from build123d import *
from build123d.topology import SkipClean

# Parameters (mm, degrees)
SKETCH_1_R               = 2.05
EXTRUDE_1_DEPTH          = 3
EXTRUDE_START            = -3
SKETCH_2_R               = 2.05
SKETCH_2_R_2             = 1.65
SKETCH_2_R_3             = 6
EXTRUDE_2_DEPTH          = 3
SKETCH_3_R               = 4
EXTRUDE_3_DEPTH          = 2
EXTRUDE_4_DEPTH          = 1.5
SKETCH_5_R               = 12.75
SKETCH_5_R_2             = 10.75
EXTRUDE_5_DEPTH          = 20
CUT_EXTRUDE_START        = -3
SKETCH_6_R               = 10.75
CUT_EXTRUDE_1_DEPTH      = 3
SKETCH_8_R               = 12.75
SKETCH_8_R_2             = 6.5
EXTRUDE_6_DEPTH          = 2
CUT_EXTRUDE_2_REACH      = 43.774
CUT_EXTRUDE_2_END_RADIUS = 12.75
SKETCH_9_W               = 4.2
SKETCH_9_H               = 6.2
SKETCH_10_W              = 14.2
SKETCH_10_H              = 10.2
SKETCH_10_W_2            = 4.2
SKETCH_10_H_2            = 6.2
EXTRUDE_9_DEPTH          = 5


with BuildPart() as part:
    # Эскиз1 → Бобышка-Вытянуть1 (new body)
    with BuildSketch(Plane.XY):
        with BuildLine():
            Line((-12.130016239, -22.05), (6.63618183, -22.05))
            ThreePointArc((6.63618183, -22.05), (7.548005274, -22.228445915), (8.47712251, -22.225976525))
            Line((8.47712251, -22.225976525), (18.824472693, -21.181334498))
            ThreePointArc((18.824472693, -21.181334498), (20.266447405, -20.813145093), (21.53617652, -20.036844583))
            Line((21.53617652, -20.036844583), (24.285575219, -17.729825148))
            ThreePointArc((24.285575219, -17.729825148), (24.812615574, -17.042972786), (25, -16.197736262))
            Line((25, -16.197736262), (25, -14.258781673))
            ThreePointArc((25, -14.258781673), (24.927604034, -13.725543744), (24.715657311, -13.230910089))
            ThreePointArc((24.715657311, -13.230910089), (23.352457929, -10.503222461), (22.419778084, -7.6))
            Line((22.419778084, -7.6), (20.113215923, -7.6))
            ThreePointArc((20.113215923, -7.6), (16.619779633, -11.410056927), (12, -13.729166034))
            Line((12, -13.729166034), (12, -17.5))
            ThreePointArc((12, -17.5), (8, -21.5), (4, -17.5))
            Line((4, -17.5), (4, -13.729166034))
            ThreePointArc((4, -13.729166034), (-6.3, 0), (4, 13.729166034))
            Line((4, 13.729166034), (4, 17.5))
            ThreePointArc((4, 17.5), (8, 21.5), (12, 17.5))
            Line((12, 17.5), (12, 13.729166034))
            ThreePointArc((12, 13.729166034), (16.619779633, 11.410056927), (20.113215923, 7.6))
            Line((20.113215923, 7.6), (22.419778084, 7.6))
            ThreePointArc((22.419778084, 7.6), (23.352457929, 10.503222461), (24.715657311, 13.230910089))
            ThreePointArc((24.715657311, 13.230910089), (24.927604034, 13.725543744), (25, 14.258781673))
            Line((25, 14.258781673), (25, 16.197736262))
            ThreePointArc((25, 16.197736262), (24.812615574, 17.042972786), (24.285575219, 17.729825148))
            Line((24.285575219, 17.729825148), (21.53617652, 20.036844583))
            ThreePointArc((21.53617652, 20.036844583), (20.266447405, 20.813145093), (18.824472693, 21.181334498))
            Line((18.824472693, 21.181334498), (8.47712251, 22.225976525))
            ThreePointArc((8.47712251, 22.225976525), (8.035899486, 22.249864338), (7.594365799, 22.232648402))
            ThreePointArc((7.594365799, 22.232648402), (5.461401325, 22.09568297), (3.324532109, 22.05))
            Line((3.324532109, 22.05), (-12.130016239, 22.05))
            ThreePointArc((-12.130016239, 22.05), (-13.477844915, 21.527618984), (-14.121593477, 20.233357861))
            ThreePointArc((-14.121593477, 20.233357861), (-14.900607263, 16.481804182), (-16.5, 13))
            Line((-16.5, 13), (-16.5, -13))
            ThreePointArc((-16.5, -13), (-14.900607263, -16.481804182), (-14.121593477, -20.233357861))
            ThreePointArc((-14.121593477, -20.233357861), (-13.477844915, -21.527618984), (-12.130016239, -22.05))
        make_face()
        with Locations((-10, -18)):
            Circle(SKETCH_1_R, mode=Mode.SUBTRACT)
        with Locations((20.855752194, -15.320888862)):
            Circle(SKETCH_1_R, mode=Mode.SUBTRACT)
        with Locations((20.855752194, 15.320888862)):
            Circle(SKETCH_1_R, mode=Mode.SUBTRACT)
        with Locations((-10, 18)):
            Circle(SKETCH_1_R, mode=Mode.SUBTRACT)
    extrude(amount=EXTRUDE_1_DEPTH)

    # Эскиз2 → Бобышка-Вытянуть2 (add)
    # profile 1 of 5: a face of its own
    with SkipClean():  # the faces are left unmerged after this step: merging them gives an invalid solid
        with BuildSketch(Plane.XY.offset(3).offset(EXTRUDE_START)):
            with Locations((20.855752194, -15.320888862)):
                Circle(SKETCH_2_R)
            with Locations((20.855752194, -15.320888862)):
                Circle(SKETCH_2_R_2, mode=Mode.SUBTRACT)
        # profile 2 of 5: a face of its own
        with BuildSketch(Plane.XY.offset(3).offset(EXTRUDE_START)):
            with Locations((-10, -18)):
                Circle(SKETCH_2_R)
            with Locations((-10, -18)):
                Circle(SKETCH_2_R_2, mode=Mode.SUBTRACT)
        # profile 3 of 5: a face of its own
        with BuildSketch(Plane.XY.offset(3).offset(EXTRUDE_START)):
            with Locations((20.855752194, 15.320888862)):
                Circle(SKETCH_2_R)
            with Locations((20.855752194, 15.320888862)):
                Circle(SKETCH_2_R_2, mode=Mode.SUBTRACT)
        # profile 4 of 5: a face of its own
        with BuildSketch(Plane.XY.offset(3).offset(EXTRUDE_START)):
            with Locations((-10, 18)):
                Circle(SKETCH_2_R)
            with Locations((-10, 18)):
                Circle(SKETCH_2_R_2, mode=Mode.SUBTRACT)
        # profile 5 of 5: a face of its own
        with BuildSketch(Plane.XY.offset(3).offset(EXTRUDE_START)):
            with BuildLine():
                Line((20.113215923, 7.6), (22.419778084, 7.6))
                ThreePointArc((22.419778084, 7.6), (22.497639732, 7.450398794), (22.573949362, 7.3))
                Line((22.573949362, 7.3), (25, 7.3))
                Line((25, 7.3), (25, -7.3))
                Line((25, -7.3), (22.573949362, -7.3))
                ThreePointArc((22.573949362, -7.3), (22.497639732, -7.450398794), (22.419778084, -7.6))
                Line((22.419778084, -7.6), (20.113215923, -7.6))
                ThreePointArc((20.113215923, -7.6), (16.619779633, -11.410056927), (12, -13.729166034))
                Line((12, -13.729166034), (12, -17.5))
                ThreePointArc((12, -17.5), (8, -13.5), (4, -17.5))
                Line((4, -17.5), (4, -13.729166034))
                ThreePointArc((4, -13.729166034), (-6.3, 0), (4, 13.729166034))
                Line((4, 13.729166034), (4, 17.5))
                ThreePointArc((4, 17.5), (8, 13.5), (12, 17.5))
                Line((12, 17.5), (12, 13.729166034))
                ThreePointArc((12, 13.729166034), (16.619779633, 11.410056927), (20.113215923, 7.6))
            make_face()
            Circle(SKETCH_2_R_3, mode=Mode.SUBTRACT)
        extrude(amount=EXTRUDE_2_DEPTH)

    # Эскиз3 → Бобышка-Вытянуть3 (add)
    # profile 1 of 2: a face of its own
    with SkipClean():  # the faces are left unmerged after this step: merging them gives an invalid solid
        with BuildSketch(Plane.XY.offset(3)):
            with BuildLine():
                Line((11.235733835, 21.947474176), (8.47712251, 22.225976525))
                ThreePointArc((8.47712251, 22.225976525), (8.035899486, 22.249864338), (7.594365799, 22.232648402))
                ThreePointArc((7.594365799, 22.232648402), (6.272890386, 22.137003862), (4.949344701, 22.076407133))
                ThreePointArc((4.949344701, 22.076407133), (7.887219492, 12.001156435), (11.235733835, 21.947474176))
            make_face()
            with Locations((8, 17.5)):
                Circle(SKETCH_3_R, mode=Mode.SUBTRACT)
        # profile 2 of 2: a face of its own
        with BuildSketch(Plane.XY.offset(3)):
            with BuildLine():
                Line((11.235733835, -21.947474176), (8.47712251, -22.225976525))
                ThreePointArc((8.47712251, -22.225976525), (8.035899486, -22.249864338), (7.594365799, -22.232648402))
                ThreePointArc((7.594365799, -22.232648402), (6.272890386, -22.137003862), (4.949344701, -22.076407133))
                ThreePointArc((4.949344701, -22.076407133), (7.887219492, -12.001156435), (11.235733835, -21.947474176))
            make_face()
            with Locations(Location((8, -17.5, 0), (0, 0, 180))):
                Circle(SKETCH_3_R, mode=Mode.SUBTRACT)
        extrude(amount=EXTRUDE_3_DEPTH)

    # Эскиз4 → Бобышка-Вытянуть4 (add)
    with SkipClean():  # the faces are left unmerged after this step: merging them gives an invalid solid
        with BuildSketch(Plane.XY.offset(5)):
            with BuildLine():
                Line((8.47712251, -22.225976525), (11.235733835, -21.947474176))
                ThreePointArc((11.235733835, -21.947474176), (7.887219492, -12.001156435), (4.949344701, -22.076407133))
                ThreePointArc((4.949344701, -22.076407133), (6.272890386, -22.137003862), (7.594365799, -22.232648402))
                ThreePointArc((7.594365799, -22.232648402), (8.035899486, -22.249864338), (8.47712251, -22.225976525))
            make_face()
            with BuildLine():
                Line((11.235733835, 21.947474176), (8.47712251, 22.225976525))
                ThreePointArc((8.47712251, 22.225976525), (8.035899486, 22.249864338), (7.594365799, 22.232648402))
                ThreePointArc((7.594365799, 22.232648402), (6.272890386, 22.137003862), (4.949344701, 22.076407133))
                ThreePointArc((4.949344701, 22.076407133), (7.887219492, 12.001156435), (11.235733835, 21.947474176))
            make_face()
        extrude(amount=EXTRUDE_4_DEPTH)

    # Эскиз5 → Бобышка-Вытянуть5 (add)
    with SkipClean():  # the faces are left unmerged after this step: merging them gives an invalid solid
        with BuildSketch(Plane.XY.offset(3)):
            Circle(SKETCH_5_R)
            Circle(SKETCH_5_R_2, mode=Mode.SUBTRACT)
        extrude(amount=EXTRUDE_5_DEPTH)

    # Эскиз6 → Вырез-Вытянуть1 (cut)
    with SkipClean():  # the faces are left unmerged after this step: merging them gives an invalid solid
        with BuildSketch(Plane.XY.offset(3).offset(CUT_EXTRUDE_START)):
            Circle(SKETCH_6_R)
        extrude(amount=CUT_EXTRUDE_1_DEPTH, mode=Mode.SUBTRACT)

    # Эскиз8 → Бобышка-Вытянуть6 (add)
    with SkipClean():  # the faces are left unmerged after this step: merging them gives an invalid solid
        with BuildSketch(Plane.XY.offset(23)):
            Circle(SKETCH_8_R)
            Circle(SKETCH_8_R_2, mode=Mode.SUBTRACT)
        extrude(amount=EXTRUDE_6_DEPTH)

    # Вырез-Вытянуть2: up to this cylinder (the profile starts inside it)
    with SkipClean():  # the faces are left unmerged after this step: merging them gives an invalid solid
        cut_extrude_2_end = Plane(origin=(0, 0, 11), z_dir=(0, 0, -1)) * Cylinder(CUT_EXTRUDE_2_END_RADIUS, 120.048, mode=Mode.PRIVATE)
        # Эскиз9 → Вырез-Вытянуть2 (cut, up to the surface)
        with BuildSketch(Plane(origin=(0, 0, 0), x_dir=(0, 0, -1), z_dir=(1, 0, 0)), mode=Mode.PRIVATE) as cut_extrude_2_sk1:
            with Locations((-8, 0)):
                Rectangle(SKETCH_9_W, SKETCH_9_H)
        cut_extrude_2_tool1 = extrude(cut_extrude_2_sk1.sketch, amount=CUT_EXTRUDE_2_REACH, mode=Mode.PRIVATE) & cut_extrude_2_end
        add(cut_extrude_2_tool1.solids().sort_by_distance((0, 0, 8))[0], mode=Mode.SUBTRACT)
        # Эскиз9 → Вырез-Вытянуть2 (cut, up to the surface)
        with BuildSketch(Plane(origin=(0, 0, 0), x_dir=(0, 0, -1), z_dir=(1, 0, 0)), mode=Mode.PRIVATE) as cut_extrude_2_sk2:
            with Locations((-14, 0)):
                Rectangle(SKETCH_9_W, SKETCH_9_H)
        cut_extrude_2_tool2 = extrude(cut_extrude_2_sk2.sketch, amount=CUT_EXTRUDE_2_REACH, mode=Mode.PRIVATE) & cut_extrude_2_end
        add(cut_extrude_2_tool2.solids().sort_by_distance((0, 0, 14))[0], mode=Mode.SUBTRACT)

    # Эскиз10 → Бобышка-Вытянуть9 (add)
    with SkipClean():  # the faces are left unmerged after this step: merging them gives an invalid solid
        with BuildSketch(Plane.ZY.offset(-10.75)):
            with Locations((11, 0)):
                Rectangle(SKETCH_10_W, SKETCH_10_H)
            with Locations((14, 0)):
                Rectangle(SKETCH_10_W_2, SKETCH_10_H_2, mode=Mode.SUBTRACT)
            with Locations((8, 0)):
                Rectangle(SKETCH_10_W_2, SKETCH_10_H_2, mode=Mode.SUBTRACT)
        extrude(amount=-EXTRUDE_9_DEPTH)


solid = part.part
Part model, mm, in its own coordinate system. A direction names the side the tool comes from. Coordinates: 2 decimals unless noted, no trailing zeros. Order: outer loops, then holes, each group sorted by start corner. A loop starts at its lowest first (then second) coordinate and runs counter-clockwise, first axis right, second up.
(1) Slice it at D-D, the plane z = 21.5. Write the cut outline in (x, y), and give its area (3 significant figures).
Check sheet entries:
outline: circle Ø25.5 at (0, 0); hole circle Ø21.5 at (0, 0)
area: 148 mm2
(2) Tool access for faces 1 (the face through (13, 0, 16.1)), 2 (the face through (25, 0, 1)), 3 (the face through (8, 18, 5)), 4 (the face through (24.93, -13.73, 1.48)): list every direction of +Z, -Z, +X, -X, +Y, -Y with a clear straight run to the whole face (end or side of a thin tool).
Check sheet entries:
face 1: +X
face 2: +Z, -Z, +X, +Y, -Y
face 3: -Z
face 4: +Z, -Z, +X
(3) Probe L1, parallel to Y at x = 11.5, z = 6; L2, parallel to Y at x = 12.5, z = 9; L3, parallel to Y at x = 20, z = 2.75. List the from-to ranges inside material, lowest first.
Check sheet entries:
L1: y = -21.74 to -13.26, -5.51 to -3.1, 3.1 to 5.51, 13.26 to 21.74
L2: y = -5.1 to -3.1, 3.1 to 5.1
L3: y = -20.92 to -16.73, -13.91 to 13.91, 16.73 to 20.92
(4) Slice it at C-C, the plane y = 2. Write the cut outline in (x, z), and give its area (3 significant figures).
Check sheet entries:
outline: (-16.5, 0) - (-10.56, 0) - (-10.56, 23) - (-6.18, 23) - (-6.18, 25) - (-12.59, 25) - (-12.59, 3) - (-16.5, 3) - close; (6.18, 23) - (10.56, 23) - (10.56, 16.1) - (15.75, 16.1) - (15.75, 18.1) - (12.59, 18.1) - (12.59, 25) - (6.18, 25) - close; (10.56, 0) - (25, 0) - (25, 3) - (12.59, 3) - (12.59, 3.9) - (15.75, 3.9) - (15.75, 5.9) - (10.56, 5.9) - close; (10.56, 10.1) - (15.75, 10.1) - (15.75, 11.9) - (10.56, 11.9) - close
area: 169 mm2
(5) Slice it at A-A, the plane x = 0. Write the cut outline in (y, z).
Check sheet entries:
outline: (-22.05, 0) - (-10.75, 0) - (-10.75, 23) - (-6.5, 23) - (-6.5, 25) - (-12.75, 25) - (-12.75, 3) - (-22.05, 3) - close; (6.5, 23) - (10.75, 23) - (10.75, 0) - (22.05, 0) - (22.05, 3) - (12.75, 3) - (12.75, 25) - (6.5, 25) - close
(6) Slice it at B-B, the plane z = 12.75. Write the cut outline in (x, y), and give its area (3 significant figures).
Check sheet entries:
outline: (10.29, -3.1) arc R10.75 cw (long way) to (10.29, 3.1) - (15.75, 3.1) - (15.75, 5.1) - (11.69, 5.1) arc R12.75 ccw (long way) to (11.69, -5.1) - (15.75, -5.1) - (15.75, -3.1) - close
area: 150 mm2
(7) Pull direction X, two halves, no side cores. Call faces 5 (the face through (-4, 22.05, 1)), 6 (the face through (-13.493, -21.514, 1.479)), 7 (the face through (23.336, 10.464, 1.479)), 8 (the face through (-5.158, -3.955, 23.986)): pulls with the +X half, pulls with the -X half, needs draft (parallel to the pull), parting line crosses it, or undercut.
Check sheet entries:
face 5: needs draft
face 6: pulls with the -X half
face 7: pulls with the +X half
face 8: undercut
(8) Pin check, flat tips, straight feed: pin 1 Ø3 at (x, z) = (-11, 14) entering from +Y; pin 2 Ø3.5 at (x, z) = (13.5, 10.5) entering from -Y; pin 3 Ø4 at (x, z) = (7, 9.5) entering from +Y. Stop position of each tip, or through.
Check sheet entries:
pin 1: stops at y = 8.5
pin 2: stops at y = -5.1
pin 3: stops at y = 11.73
